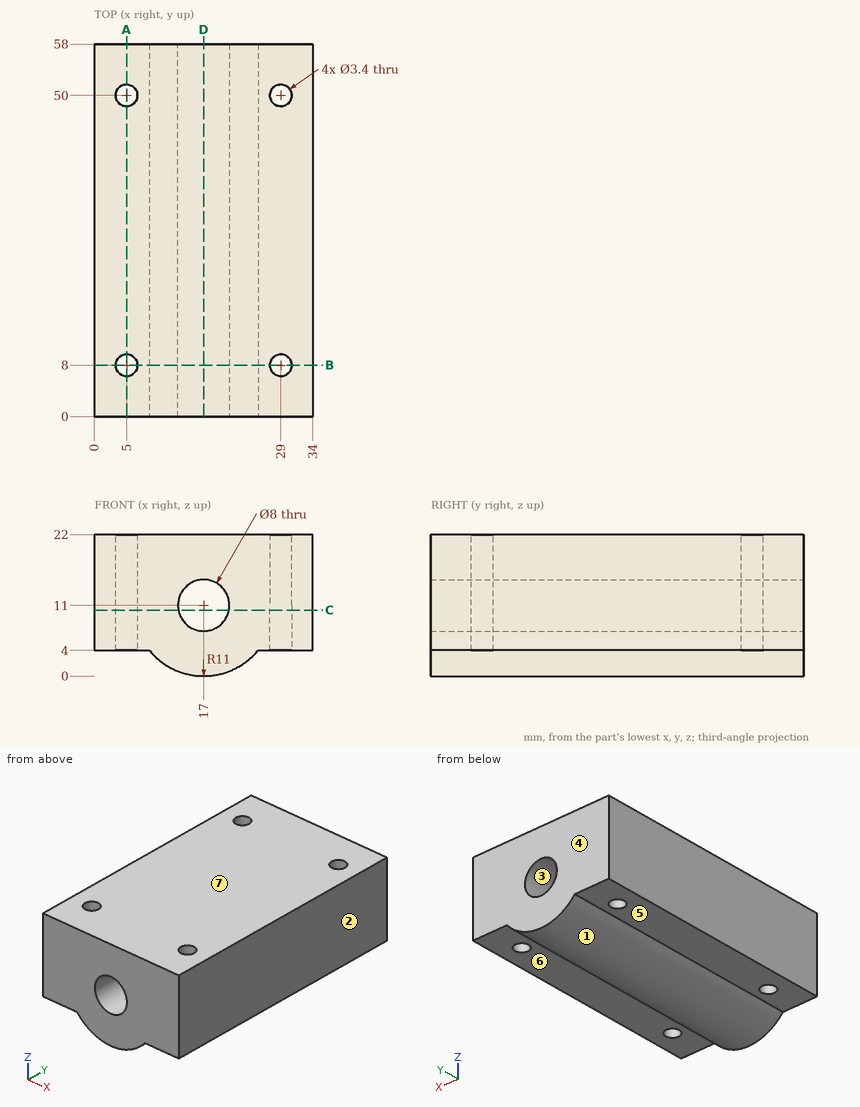
Job drawing, mm, ordinate dimensions from the low corner. One solid piece. A direction names the side the tool comes from. Coordinates: 2 decimals unless noted, no trailing zeros. Order: outer loops, then holes, each group sorted by start corner. A loop starts at its lowest first (then second) coordinate and runs counter-clockwise, first axis right, second up. Notation, with made-up numbers: M 18.5,62 L 65.5,62 A19 cw 65.5,77 Z; hole C 16,67 d8. An arc over 180 degrees is marked long. Answer as CSV lines item,"result".
(1) Wall check: line 1 along Y through (x, z) = (29, 15); line 2 along X through (y, z) = (8, 17.75); line 3 along X through (y, z) = (48.5, 5.5). Give the ranges that are in metal, low to high.
Geometry says:
line 1,"y = 0 to 6.3, 9.7 to 48.3, 51.7 to 58"
line 2,"x = 0 to 3.3, 6.7 to 27.3, 30.7 to 34"
line 3,"x = 0 to 4.2, 5.8 to 28.2, 29.8 to 34"
(2) Band-saw the part on B-B, the plane y = 8. List the corners of the cut face in (x, z), then the cut area to 3 significant figures.
Geometry says:
outline,"M 0,4 L 3.3,4 L 3.3,22 L 0,22 Z; M 6.7,4 L 8.51,4 A11 ccw 25.49,4 L 27.3,4 L 27.3,22 L 6.7,22 Z; M 30.7,4 L 34,4 L 34,22 L 30.7,22 Z; hole C 17,11 d8"
area,"487 mm2"
(3) Band-saw the part on A-A, the plane x = 5. List the corners of the cut face in (y, z).
Geometry says:
outline,"M 0,4 L 6.3,4 L 6.3,22 L 0,22 Z; M 9.7,4 L 48.3,4 L 48.3,22 L 9.7,22 Z; M 51.7,4 L 58,4 L 58,22 L 51.7,22 Z"
(4) Flat gauge pins, fed straight in: pin 1 (9.5 mm diameter, centred on x = 30.5, y = 21, fed in from -Z); pin 2 (3 mm diameter, centred on x = 5, y = 50, fed in from +Z). Where does each tip first touch, or does it go through?
Geometry says:
pin 1,"stops at z = 4"
pin 2,"passes through"
(5) 3-axis set-ups, long thin cutter, end or side, ignore diameter. For the marked faces 5, 6 and 7: which of +Z, -Z, +X, -X, +Y, -Y reach the whole face in a straight line?
Geometry says:
face 5,"-Z, -X, +Y, -Y"
face 6,"-Z, +X, +Y, -Y"
face 7,"+Z, +X, -X, +Y, -Y"
(6) Pull direction X, two halves, no side cores. Call the marked faces 1, 2, 3 and 4: +X half, -X half, draft (parallel to the pull), parting line (faces both ways), or undercut.
Geometry says:
face 1,"parting line"
face 2,"+X half"
face 3,"undercut"
face 4,"draft"
(7) Band-saw the part on D-D, the plane x = 17. List the corners of the cut face in (y, z), then the cut area to 3 significant figures.
Geometry says:
outline,"M 0,0 L 58,0 L 58,7 L 0,7 Z; M 0,15 L 58,15 L 58,22 L 0,22 Z"
area,"812 mm2"
(8) Band-saw the part on C-C, the plane z = 10.25. List the corners of the cut face in (x, y).
Geometry says:
outline,"M 0,0 L 13.07,0 L 13.07,58 L 0,58 Z; M 20.93,0 L 34,0 L 34,58 L 20.93,58 Z; hole C 5,8 d3.4; hole C 5,50 d3.4; hole C 29,8 d3.4; hole C 29,50 d3.4"
